Check sheet for the drawn part. Datum: minimum x, y, z corner. Units: mm. Round coordinates to 2 decimals unless told otherwise and drop trailing zeros. Order: outer loops, then holes, each group sorted by start corner. A loop starts at its lowest first (then second) coordinate and runs counter-clockwise, first axis right, second up. Notation, with made-up numbers: (32, -18.5) -> (66, -18.5) arc R24 cw to (66, 8.5) -> close; hole circle Ø8 at (30.5, 14). An arc over 180 degrees is marked (long way). Answer in a Markdown table with one row per item.
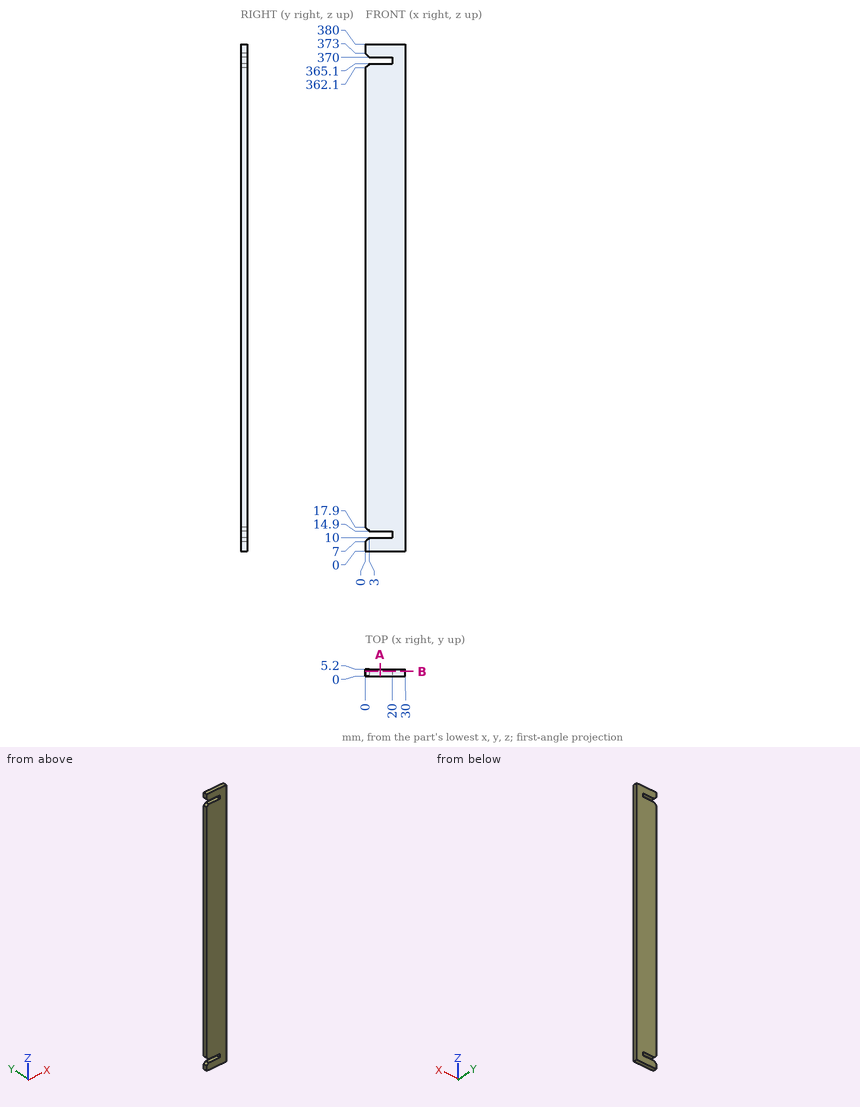
(1) Scan lines: probe 1 along Z at (x, y) = (10, 2.75); probe 2 along Z at (x, y) = (2, 4.3). Record each from-to range of solid material in increasing order. Write a range as from..to.
Solutions:
| item | result |
|---|---|
| probe 1 | 0..10, 14.9..365.1, 370..380 |
| probe 2 | 0..9, 15.9..364.1, 371..380 |
(2) Depth check by flat-ended pin: pin 1 Ø1 at (x, y) = (24.5, 1.5) entering from -Z. Enter the tip coordinate at first touch or a pass-through.
Solutions:
| item | result |
|---|---|
| pin 1 | z = 0 |
(3) Section check B-B on y = 3.45. Record the boundary of the cut face in (x, z), plus the area to 3 significant figures.
Solutions:
| item | result |
|---|---|
| outline | (0, 0) -> (30, 0) -> (30, 380) -> (0, 380) -> (0, 373) -> (3, 370) -> (20, 370) -> (20, 365.1) -> (3, 365.1) -> (0, 362.1) -> (0, 17.9) -> (3, 14.9) -> (20, 14.9) -> (20, 10) -> (3, 10) -> (0, 7) -> close |
| area | 11,200 mm^2 |
(4) Section check A-A on x = 11. Record the boundary of the cut face in (y, z), plus the area to 3 significant figures.
Solutions:
| item | result |
|---|---|
| outline | (0, 0) -> (5.2, 0) -> (5.2, 10) -> (0, 10) -> close; (0, 14.9) -> (5.2, 14.9) -> (5.2, 365.1) -> (0, 365.1) -> close; (0, 370) -> (5.2, 370) -> (5.2, 380) -> (0, 380) -> close |
| area | 1,930 mm^2 |
